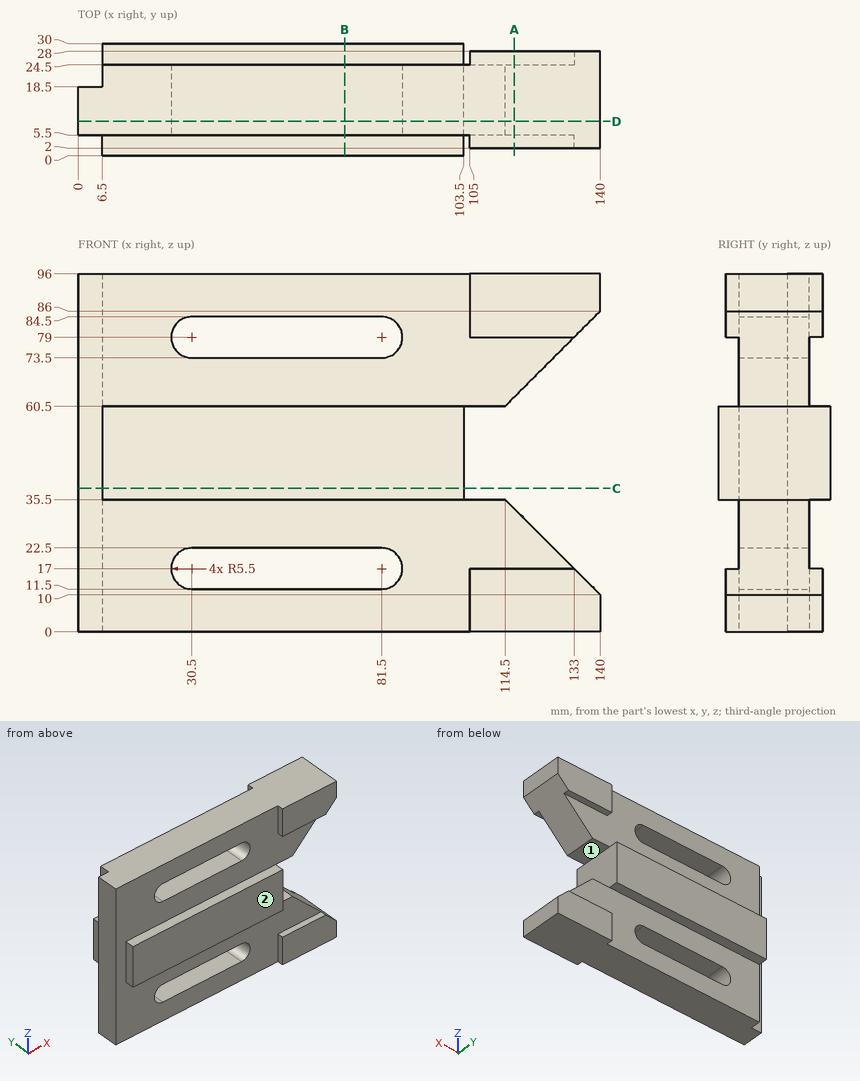
Check sheet for the drawn part. Datum: minimum x, y, z corner. Units: mm. A direction names the side the tool comes from. Round coordinates to 2 decimals unless told otherwise and drop trailing zeros. Order: outer loops, then holes, each group sorted by start corner. A loop starts at its lowest first (then second) coordinate and runs counter-clockwise, first axis right, second up.
1) Section check A-A (x = 117). Record the boundary of the cut face in (y, z), and give its area (3 significant figures).
2) Scan lines: line 1 (Z direction, x = 32, y = 15.5); line 2 (Z direction, x = 109, y = 17.75); line 3 (Z direction, x = 28, y = 12.75). Record each from-to range of solid material in increasing order.
3) Section check B-B (x = 71.5). Record the boundary of the cut face in (y, z), and give its area (3 significant figures).
4) Section check D-D (y = 9.25). Record the boundary of the cut face in (x, z), and give its area (3 significant figures).
5) Tool access check on the marked faces 1 and 2. Record the directions out of +Z, -Z, +X, -X, +Y, -Y that give a thin tool (end or side, any length) a straight path to the whole face; none if there is none.
6) Section check C-C (z = 38.5). Record the boundary of the cut face in (x, y), and give its area (3 significant figures).
7) Go/stop test with flat-tipped pins: pin 1 Ø1.8 at (y, z) = (4, 91) entering from -X; pin 2 Ø3 at (x, z) = (120.5, 68) entering from +Y; pin 3 Ø5 at (x, z) = (125, 9) entering from +Y. Record where each tip stops, or that it passes through.
Result:
1. outline: (2, 0) - (28, 0) - (28, 17) - (24.5, 17) - (24.5, 33) - (5.5, 33) - (5.5, 17) - (2, 17) - close; (2, 79) - (5.5, 79) - (5.5, 63) - (24.5, 63) - (24.5, 79) - (28, 79) - (28, 96) - (2, 96) - close
1. area: 1,490 mm2
2. line 1: z = 0 to 11.5, 22.5 to 73.5, 84.5 to 96
2. line 2: z = 0 to 35.5, 60.5 to 96
2. line 3: z = 0 to 12.1, 21.9 to 74.1, 83.9 to 96
3. outline: (0, 35.5) - (5.5, 35.5) - (5.5, 22.5) - (24.5, 22.5) - (24.5, 35.5) - (30, 35.5) - (30, 60.5) - (24.5, 60.5) - (24.5, 73.5) - (5.5, 73.5) - (5.5, 60.5) - (0, 60.5) - close; (5.5, 0) - (24.5, 0) - (24.5, 11.5) - (5.5, 11.5) - close; (5.5, 84.5) - (24.5, 84.5) - (24.5, 96) - (5.5, 96) - close
3. area: 1,680 mm2
4. outline: (0, 0) - (140, 0) - (140, 10) - (114.5, 35.5) - (103.5, 35.5) - (103.5, 60.5) - (114.5, 60.5) - (140, 86) - (140, 96) - (0, 96) - close; hole (30.5, 11.5) - (81.5, 11.5) arc R5.5 ccw to (81.5, 22.5) - (30.5, 22.5) arc R5.5 ccw to start; hole (30.5, 73.5) - (81.5, 73.5) arc R5.5 ccw to (81.5, 84.5) - (30.5, 84.5) arc R5.5 ccw to start
4. area: 10,600 mm2
5. face 1: +X, +Y, -Y
5. face 2: +Z, -Z, +X, -X, -Y
6. outline: (0, 5.5) - (6.5, 5.5) - (6.5, 0) - (103.5, 0) - (103.5, 30) - (6.5, 30) - (6.5, 18.5) - (0, 18.5) - close
6. area: 2,990 mm2
7. pin 1: stops at x = 105
7. pin 2: stops at y = 24.5
7. pin 3: stops at y = 28
